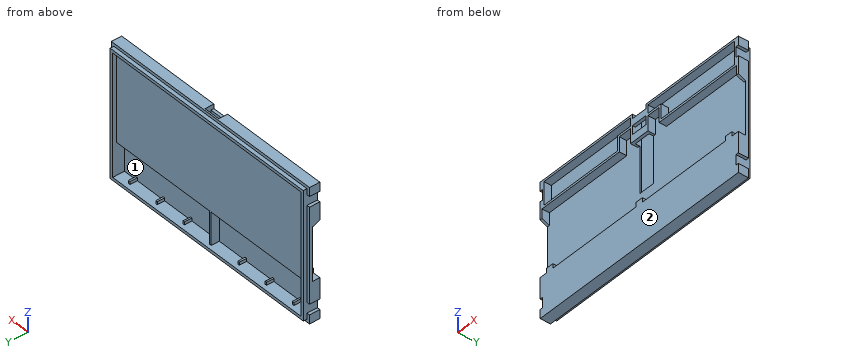
from build123d import *

# Parameters (mm, degrees)
SKETCH_1_W                 = 159.5
SKETCH_1_H                 = 90.2
EXTRUDE_1_DEPTH            = 9.5
SKETCH_2_W                 = 163.5
SKETCH_2_H                 = 94.2
SKETCH_2_W_2               = 155.5
SKETCH_2_H_2               = 86.2
CUT_EXTRUDE_1_DEPTH        = 2.5
SKETCH_3_W                 = 151.5
SKETCH_3_H                 = 82.2
CUT_EXTRUDE_2_DEPTH        = 2.5
SKETCH_4_W                 = 151.5
SKETCH_4_H                 = 22
CUT_EXTRUDE_3_DEPTH        = 5.5
SKETCH_5_W                 = 1.2
SKETCH_5_H                 = 22
EXTRUDE_2_DEPTH            = 5.5
SKETCH_7_W                 = 1.2
SKETCH_7_H                 = 2
EXTRUDE_4_DEPTH            = 5
PATTERN_LINEAR_1_COUNT     = 4
PATTERN_LINEAR_1_PITCH     = 22
PATTERN_LINEAR_1_COL_COUNT = 4
PATTERN_LINEAR_1_COL_PITCH = 22
SKETCH_8_W                 = 2
SKETCH_8_H                 = 7
CUT_EXTRUDE_4_DEPTH        = 92.886193196
CUT_EXTRUDE_5_DEPTH        = 167.025630551
EXTRUDE_5_DEPTH            = 2.5
PATTERN_LINEAR_2_COUNT     = 2
PATTERN_LINEAR_2_PITCH     = 72
PATTERN_LINEAR_2_COL_COUNT = 2
PATTERN_LINEAR_2_COL_PITCH = 72
SKETCH_11_W                = 153.5
SKETCH_11_H                = 15.6
CUT_EXTRUDE_6_DEPTH        = 5
SKETCH_12_W                = 156.5
SKETCH_12_H                = 10
CUT_EXTRUDE_7_DEPTH        = 5
SKETCH_13_W                = 32
SKETCH_13_H                = 10
CUT_EXTRUDE_8_DEPTH        = 5
EXTRUDE_6_DEPTH            = 5
SKETCH_15_W                = 14
SKETCH_15_H                = 18.6
EXTRUDE_7_DEPTH            = 5
SKETCH_16_W                = 11
SKETCH_16_H                = 6
SKETCH_16_H_2              = 5
CUT_EXTRUDE_9_DEPTH        = 5
SKETCH_17_W                = 11
SKETCH_17_H                = 4
CUT_EXTRUDE_10_DEPTH       = 50


with BuildPart() as part:
    # Эскиз1 → Бобышка-Вытянуть1 (new body)
    with BuildSketch(Plane(origin=(0, 0, 0), x_dir=(1, 0, 0), z_dir=(0, 1, 0))):
        Rectangle(SKETCH_1_W, SKETCH_1_H)
    extrude(amount=EXTRUDE_1_DEPTH)

    # Эскиз2 → Вырез-Вытянуть1 (cut)
    with BuildSketch(Plane(origin=(0, 9.5, 0), x_dir=(1, 0, 0), z_dir=(0, 1, 0))):
        Rectangle(SKETCH_2_W, SKETCH_2_H)
        Rectangle(SKETCH_2_W_2, SKETCH_2_H_2, mode=Mode.SUBTRACT)
    extrude(amount=-CUT_EXTRUDE_1_DEPTH, mode=Mode.SUBTRACT)

    # Эскиз3 → Вырез-Вытянуть2 (cut)
    with BuildSketch(Plane(origin=(0, 9.5, 0), x_dir=(1, 0, 0), z_dir=(0, 1, 0))):
        Rectangle(SKETCH_3_W, SKETCH_3_H)
    extrude(amount=-CUT_EXTRUDE_2_DEPTH, mode=Mode.SUBTRACT)

    # Эскиз4 → Вырез-Вытянуть3 (cut)
    with BuildSketch(Plane(origin=(0, 7, 0), x_dir=(1, 0, 0), z_dir=(0, 1, 0))):
        with Locations((0, 30.1)):
            Rectangle(SKETCH_4_W, SKETCH_4_H)
    extrude(amount=-CUT_EXTRUDE_3_DEPTH, mode=Mode.SUBTRACT)

    # Эскиз5 → Бобышка-Вытянуть2 (add)
    with BuildSketch(Plane(origin=(0, 1.5, 0), x_dir=(1, 0, 0), z_dir=(0, 1, 0))):
        with Locations((0, 30.1)):
            Rectangle(SKETCH_5_W, SKETCH_5_H)
    extrude(amount=EXTRUDE_2_DEPTH)

    # Эскиз7 → Бобышка-Вытянуть4 (add)
    with BuildSketch(Plane(origin=(0, 1.5, 0), x_dir=(1, 0, 0), z_dir=(0, 1, 0))):
        with Locations((0, 40.1)):
            Rectangle(SKETCH_7_W, SKETCH_7_H)
    extrude_4 = extrude(amount=EXTRUDE_4_DEPTH)

    # Линейный массив1: Бобышка-Вытянуть4 ×4
    with Locations(*[(-i * PATTERN_LINEAR_1_PITCH, 0, 0) for i in range(1, PATTERN_LINEAR_1_COUNT)]):
        add(extrude_4)

    # Линейный массив1 col: Бобышка-Вытянуть4 ×4
    with Locations(*[(i * PATTERN_LINEAR_1_COL_PITCH, 0, 0) for i in range(1, PATTERN_LINEAR_1_COL_COUNT)]):
        add(extrude_4)

    # Эскиз8 → Вырез-Вытянуть4 (cut, through all)
    with BuildSketch(Plane(origin=(0, 7, 0), x_dir=(1, 0, 0), z_dir=(0, 1, 0))):
        with Locations((78.75, 35.6)):
            Rectangle(SKETCH_8_W, SKETCH_8_H)
        with Locations((78.75, -35.6)):
            Rectangle(SKETCH_8_W, SKETCH_8_H)
    cut_extrude_4 = extrude(amount=-CUT_EXTRUDE_4_DEPTH, mode=Mode.SUBTRACT)

    # Зеркальное отражение1: Вырез-Вытянуть4 across plane
    add(cut_extrude_4.mirror(Plane(origin=(0, 0, 0), x_dir=(0, 0, 1), z_dir=(1, 0, 0))), mode=Mode.SUBTRACT)

    # Эскиз9 → Вырез-Вытянуть5 (cut, through all)
    with BuildSketch(Plane(origin=(79.75, 0, 0), x_dir=(0, 0, -1), z_dir=(1, 0, 0))):
        Polygon((-21, -2), (-18, 5), (18, 5), (18, -2), align=None)
    extrude(amount=-CUT_EXTRUDE_5_DEPTH, mode=Mode.SUBTRACT)

    # Эскиз10 → Бобышка-Вытянуть5 (add, symmetric)
    with BuildSketch(Plane(origin=(0, 0, 0), x_dir=(0, 0, -1), z_dir=(1, 0, 0))):
        Polygon((18, 0), (15, 0), (15, 2.5), (17.6, 3.6), (17.6, 5.1), (18.1, 5.1), (18.1, 0), align=None)
    extrude_5 = extrude(amount=EXTRUDE_5_DEPTH, both=True)

    # Линейный массив2: Бобышка-Вытянуть5 ×2
    with Locations(*[(i * PATTERN_LINEAR_2_PITCH, 0, 0) for i in range(1, PATTERN_LINEAR_2_COUNT)]):
        add(extrude_5)

    # Линейный массив2 col: Бобышка-Вытянуть5 ×2
    with Locations(*[(-i * PATTERN_LINEAR_2_COL_PITCH, 0, 0) for i in range(1, PATTERN_LINEAR_2_COL_COUNT)]):
        add(extrude_5)

    # Эскиз11 → Вырез-Вытянуть6 (cut)
    with BuildSketch(Plane.XZ):
        with Locations((0, 35.8)):
            Rectangle(SKETCH_11_W, SKETCH_11_H)
    extrude(amount=-CUT_EXTRUDE_6_DEPTH, mode=Mode.SUBTRACT)

    # Эскиз12 → Вырез-Вытянуть7 (cut)
    with BuildSketch(Plane.XZ):
        with Locations((0, 21.5)):
            Rectangle(SKETCH_12_W, SKETCH_12_H)
    extrude(amount=-CUT_EXTRUDE_7_DEPTH, mode=Mode.SUBTRACT)

    # Эскиз13 → Вырез-Вытянуть8 (cut)
    with BuildSketch(Plane.XZ):
        with Locations((0, 28.6)):
            Rectangle(SKETCH_13_W, SKETCH_13_H)
    extrude(amount=-CUT_EXTRUDE_8_DEPTH, mode=Mode.SUBTRACT)

    # Эскиз14 → Бобышка-Вытянуть6 (add)
    with BuildSketch(Plane.XZ.offset(-5)):
        Polygon((-16, 28), (-16, 36.5), (16, 36.5), (16, 28), (17.5, 28), (17.5, 38), (-17.5, 38), (-17.5, 28), align=None)
    extrude(amount=EXTRUDE_6_DEPTH)

    # Эскиз15 → Бобышка-Вытянуть7 (add)
    with BuildSketch(Plane.XZ.offset(-5)):
        with Locations((0, 35.8)):
            Rectangle(SKETCH_15_W, SKETCH_15_H)
    extrude(amount=EXTRUDE_7_DEPTH)

    # Эскиз16 → Вырез-Вытянуть9 (cut)
    with BuildSketch(Plane.XZ):
        with Locations((0, 34.5)):
            Rectangle(SKETCH_16_W, SKETCH_16_H)
        with Locations((0, 44.6)):
            Rectangle(SKETCH_16_W, SKETCH_16_H_2)
    extrude(amount=-CUT_EXTRUDE_9_DEPTH, mode=Mode.SUBTRACT)

    # Эскиз17 → Вырез-Вытянуть10 (cut)
    with BuildSketch(Plane.XY.offset(45.1)):
        with Locations((0, 4)):
            Rectangle(SKETCH_17_W, SKETCH_17_H)
    extrude(amount=-CUT_EXTRUDE_10_DEPTH, mode=Mode.SUBTRACT)


solid = part.part
Verification items for the finished model (mm, model axes). Face numbers are marked on the shaded views. Give positions to 0.01 mm unless a question says otherwise; leave off trailing zeros. Loops run counter-clockwise (first coordinate to the right, second up) from the corner with the lowest first, then second, coordinate; pieces in that order, holes last.
1) Depth check by flat-ended pin: pin 1 Ø1.5 at (y, z) = (8.5, -4.5) entering from -X; pin 2 Ø3.5 at (y, z) = (1.5, -16) entering from -X; pin 3 Ø8 at (x, z) = (-37, 12.5) entering from -Y. Enter the tip coordinate at first touch or a pass-through.
2) Sectioned sample at B-B, the plane z = 4.5. Enter the section's corners in (x, y), then the cut area to 3 significant figures.
3) Sectioned sample at A-A, the plane x = -58. Enter the section's corners in (y, z), then the cut area to 3 significant figures.
4) Draft check along X on the marked faces 1 and 2. Enter one of: pulls with the +X half, pulls with the -X half, needs draft (parallel to the pull), parting line crosses it, or undercut.
5) Thickness scan on line 1 along X through (y, z) = (2.75, 30); line 2 along X through (y, z) = (5.25, -24.5); line 3 along Z through (x, y) = (-48.5, 1). Record the ranges inside material, lowest first.
Answers:
1. pin 1: stops at x = -77.75
1. pin 2: stops at x = -74.5
1. pin 3: stops at y = 5
2. outline: (-79.75, 5) - (-5.5, 5) - (-5.5, 6) - (5.5, 6) - (5.5, 5) - (79.75, 5) - (79.75, 7) - (77.75, 7) - (77.75, 9.5) - (75.75, 9.5) - (75.75, 7) - (-75.75, 7) - (-75.75, 9.5) - (-77.75, 9.5) - (-77.75, 7) - (-79.75, 7) - close
2. area: 318 mm2
3. outline: (0, -45.1) - (7, -45.1) - (7, -43.1) - (9.5, -43.1) - (9.5, -41.1) - (1.5, -41.1) - (1.5, -19.1) - (7, -19.1) - (7, 41.1) - (9.5, 41.1) - (9.5, 43.1) - (7, 43.1) - (7, 45.1) - (0, 45.1) - (0, 43.6) - (5, 43.6) - (5, 28) - (0, 28) - (0, 26.5) - (5, 26.5) - (5, -18) - (0, -18) - close
3. area: 220 mm2
4. face 1: undercut
4. face 2: needs draft
5. line 1: x = -79.75 to -76.75, -17.5 to -16, -7 to -5.5, 5.5 to 7, 16 to 17.5, 76.75 to 79.75
5. line 2: x = -79.75 to -75.75, -0.6 to 0.6, 75.75 to 79.75
5. line 3: z = -45.1 to -18, 26.5 to 28, 43.6 to 45.1
